```python
from build123d import *

# Parameters (mm, degrees)
BOSS_EXTRUDE1_DEPTH = 1
BOSS_EXTRUDE2_DEPTH = 7
SKETCH3_R           = 1.25
CUT_EXTRUDE1_DEPTH  = 7
BOSS_EXTRUDE3_DEPTH = 50
BOSS_EXTRUDE4_DEPTH = 1
SKETCH6_W           = 55.65
SKETCH6_H           = 1
BOSS_EXTRUDE5_DEPTH = 0.441482
CUT_EXTRUDE2_REACH  = 21.75
SKETCH7_W           = 0.87
SKETCH7_H           = 1


with BuildPart() as part:
    # Sketch1 → Boss-Extrude1 (new body)
    with BuildSketch(Plane.XY):
        Polygon((-28.25, -16.96), (-28.25, 16.96), (28.25, 16.96), (28.25, 2.54), (25.25, 2.54), (25.25, -2.46), (28.25, -2.46), (28.25, -9.46), (25.25, -9.46), (25.25, -14.46), (28.25, -14.46), (28.25, -16.96), align=None)
    extrude(amount=BOSS_EXTRUDE1_DEPTH)

    # Sketch2 → Boss-Extrude2 (add)
    with BuildSketch(Plane.XZ.offset(9.46)):
        with BuildLine():
            Line((28.25, 1), (31.25, 1))
            ThreePointArc((31.25, 1), (28.25, 4), (25.25, 1))
            Line((25.25, 1), (28.25, 1))
        make_face()
    extrude(amount=-BOSS_EXTRUDE2_DEPTH)

    # Sketch3 → Cut-Extrude1 (cut)
    with BuildSketch(Plane(origin=(0, -2.46, 0), x_dir=(1, 0, 0), z_dir=(0, 1, 0))):
        with Locations((28.25, -2.4)):
            Circle(SKETCH3_R)
    extrude(amount=-CUT_EXTRUDE1_DEPTH, mode=Mode.SUBTRACT)

    # Sketch4 → Boss-Extrude3 (add)
    with BuildSketch(Plane.ZY.offset(28.25)):
        Polygon((1, 13.04), (3.5, 10.54), (3.5, -14.46), (1, -16.96), align=None)
    extrude(amount=-BOSS_EXTRUDE3_DEPTH)



with BuildPart() as body_2:
    # Sketch5 → Boss-Extrude4 (new body)
    with BuildSketch(Plane(origin=(0, 7.593598631, 8.433545673), x_dir=(-1, 0, 0), z_dir=(0, 0.669130606, 0.743144825))):
        Polygon((28.25, -11.934605634), (28.25, -39.514605634), (11.95, -39.514605634), (-27.4, -15.434605634), (-27.4, -11.934605634), align=None)
    extrude(amount=-BOSS_EXTRUDE4_DEPTH)


with BuildPart() as part_1:
    add(part.part)

    add(body_2.part)  # Boss-Extrude5 merges body 2
    # Sketch6 → Boss-Extrude5 (add)
    with BuildSketch(Plane(origin=(0, 8.869140421, -7.985809904), x_dir=(1, 0, 0), z_dir=(0, -0.743144825, 0.669130606))):
        with Locations((-0.425, 10.848455084)):
            Rectangle(SKETCH6_W, SKETCH6_H)
    extrude(amount=BOSS_EXTRUDE5_DEPTH)

    # Cut-Extrude2: up to this face of the body (flat: up to its plane)
    cut_extrude2_end = Plane(part_1.part.faces().sort_by_distance((-6.843835743, 23.936811471, -7.627581995))[0])
    # Sketch7 → Cut-Extrude2 (cut, up to the picked face)
    with BuildSketch(Plane.XY.offset(1), mode=Mode.PRIVATE) as cut_extrude2_sk1:
        with Locations((27.815, 16.46)):
            Rectangle(SKETCH7_W, SKETCH7_H)
    cut_extrude2_tool1 = split(extrude(cut_extrude2_sk1.sketch, amount=-CUT_EXTRUDE2_REACH, mode=Mode.PRIVATE), bisect_by=cut_extrude2_end, keep=Keep.BOTH, mode=Mode.PRIVATE)
    add(cut_extrude2_tool1.solids().sort_by_distance((27.815, 16.46, 1))[0], mode=Mode.SUBTRACT)


solid = part_1.part
```
For this review, take the finished solid that the model builds, in its own axes (mm). A direction names the side the tool comes from. Coordinates: 2 decimals unless noted, no trailing zeros. Loops run counter-clockwise (first coordinate to the right, second up) from the corner with the lowest first, then second, coordinate; pieces in that order, holes last. Notation, with made-up numbers: (72.25, 81) -> (104.25, 81) arc R15 ccw to (104.25, 100) -> close; hole circle Ø2 at (86.5, 78). An arc over 180 degrees is marked (long way). Return JSON: item names as keys, results as strings. Group by question number.
(1) To check wall thickness, follow L1, parallel to X at y = -6.75, z = 2.4; L2, parallel to Z at x = -22.5, y = 8.5; L3, parallel to Z at x = 28, y = -4. State the ranges of each line that lie inside material, in increasing order.
(2) Tool access review of faces 1 (the flat face through (21.75, -2, 2)), 2 (the flat face through (-4, -2, 3.5)), 3 (the flat face through (28, -9.46, 1)): name each direction out of +Z, -Z, +X, -X, +Y, -Y from which nothing blocks a thin tool from reaching the whole face with its end or side.
(3) Consider section B-B, the plane z = 2.4. Give the boundary of the cut face in (x, y), plus the area to 3 significant figures.
(4) For pin 1 Ø4.5 at (x, z) = (28.5, 2) entering from -Y; pin 2 Ø0.5 at (y, z) = (-11.5, 0.5) entering from +X; pin 3 Ø5 at (x, y) = (-4, 0.5) entering from -Z; pin 4 Ø10 at (x, y) = (14.5, 24) entering from +Z, all flat-tipped, find the tip position at first contact; note any pin that passes through.
(5) Consider section D-D, the plane z = -8.25. Give the boundary of the cut face in (x, y), plus the area to 3 significant figures.
(6) Consider section A-A, the plane y = -8. Give the boundary of the cut face in (x, z), plus the area to 3 significant figures.
(7) Consider section C-C, the plane x = 11. Give the boundary of the cut face in (y, z).
(8) Mouldability with a two-part tool opening along Z and no side actions: class faces 4 (the flat face through (-3.6, 11.81, 2.23)), 5 (the flat face through (-28.25, 5.1, 0.5)), 6 (the flat face through (0, 0, 0)), 7 (the cylindrical face through (29.405, -5.911, 2.879)) as pulls with the +Z half, pulls with the -Z half, needs draft (parallel to the pull), parting line crosses it, or undercut.
Results below:
{
 "1": {"L1": "x = -28.25 to 21.75, 25.6 to 27, 29.5 to 30.9", "L2": "z = 0 to 3.5", "L3": "z = 0 to 1.18, 3.62 to 3.99"},
 "2": {"face 1": "+Z, +Y, -Y", "face 2": "+Z, -X, +Y, -Y", "face 3": "+Z, -Z, +X"},
 "3": {"outline": "(-28.25, -15.56) -> (21.75, -15.56) -> (21.75, 11.64) -> (-28.25, 11.64) -> close; (25.6, -9.46) -> (27, -9.46) -> (27, -2.46) -> (25.6, -2.46) -> close; (29.5, -9.46) -> (30.9, -9.46) -> (30.9, -2.46) -> (29.5, -2.46) -> close", "area": "1,380 mm2"},
 "4": {"pin 1": "stops at y = -16.96", "pin 2": "stops at x = 25.25", "pin 3": "stops at z = 0", "pin 4": "stops at z = -1.84"},
 "5": {"outline": "(-28.25, 24.63) -> (13.69, 24.63) -> (11.88, 26.12) -> (-28.25, 26.12) -> close", "area": "61.3 mm2"},
 "6": {"outline": "(-28.25, 0) -> (28.25, 0) -> (28.25, 1) -> (31.25, 1) arc R3 ccw to (25.25, 1) -> (21.75, 1) -> (21.75, 3.5) -> (-28.25, 3.5) -> close; hole circle Ø2.5 at (28.25, 2.4)", "area": "191 mm2"},
 "7": {"outline": "(-16.96, 0) -> (15.47, 0) -> (25.85, -9.35) -> (26.52, -8.61) -> (16.96, 0) -> (16.96, 1) -> (13.04, 1) -> (10.54, 3.5) -> (-14.46, 3.5) -> (-16.96, 1) -> close"},
 "8": {"face 4": "pulls with the +Z half", "face 5": "needs draft", "face 6": "pulls with the -Z half", "face 7": "undercut"}
}
